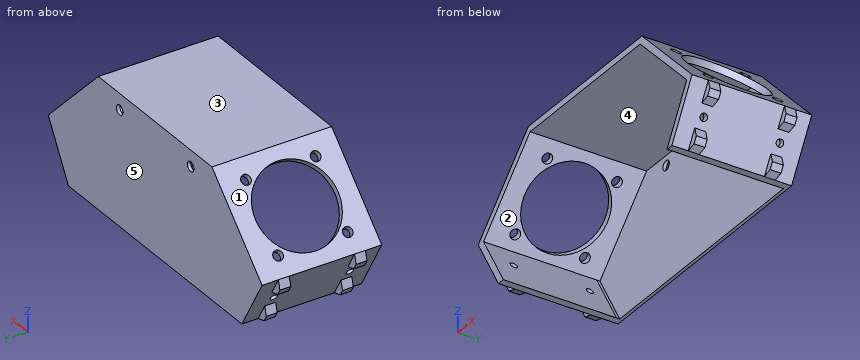
from build123d import *

# Parameters (mm, degrees)
BOSS_EXTRUDE1_DEPTH      = 55
SHELL1_T                 = -3
CUT_EXTRUDE1_REACH       = 167.077
SKETCH2_R                = 19
SKETCH2_R_2              = 2.25
CUT_EXTRUDE2_REACH       = 170.904
SKETCH3_R                = 1.65
SKETCH4_W                = 9.228601628
SKETCH4_H                = 5
BOSS_EXTRUDE2_DEPTH      = 3
CHAMFER1_SIZE            = 3
CHAMFER1_OF_MIRROR2_SIZE = 3
SKETCH5_R                = 2.25
CUT_EXTRUDE3_DEPTH       = 147.36190521
CUT_EXTRUDE4_DEPTH       = 1.5


with BuildPart() as part:
    # Sketch1 → Boss-Extrude1 (new body)
    with BuildSketch(Plane(origin=(0, 0, 0), x_dir=(1, 0, 0), z_dir=(0, 1, 0))):
        Polygon((40.050177105, -112), (-40.050177105, -112), (-75.405516164, -76.644660941), (-61.176914536, -52), (61.176914536, -52), (75.405516164, -76.644660941), align=None)
    extrude(amount=BOSS_EXTRUDE1_DEPTH)

    # Shell1
    shell1_openings = [part.faces().sort_by_distance(p)[0] for p in [
        (0, 27.5, 52),
        (0, 0, 79.968655268),
    ]]
    offset(amount=SHELL1_T, openings=shell1_openings, kind=Kind.INTERSECTION)

    # Sketch2 → Cut-Extrude1 (cut, up to next)
    with BuildSketch(Plane(origin=(76.025088553, 0, 76.025088553), x_dir=(0.7071067811865462, 0, -0.7071067811865488), z_dir=(0.7071067811865488, 0, 0.7071067811865462)), mode=Mode.PRIVATE) as cut_extrude1_sk1:
        with Locations((-25.876207674, 27.5)):
            Circle(SKETCH2_R)
    cut_extrude1_tool1 = extrude(cut_extrude1_sk1.sketch, amount=-CUT_EXTRUDE1_REACH, mode=Mode.PRIVATE) & part.part
    # Sketch2 → Cut-Extrude1 (cut, up to next)
    with BuildSketch(Plane(origin=(76.025088553, 0, 76.025088553), x_dir=(0.7071067811865462, 0, -0.7071067811865488), z_dir=(0.7071067811865488, 0, 0.7071067811865462)), mode=Mode.PRIVATE) as cut_extrude1_sk2:
        with Locations((-41.876207674, 11.5)):
            Circle(SKETCH2_R_2)
    cut_extrude1_tool2 = extrude(cut_extrude1_sk2.sketch, amount=-CUT_EXTRUDE1_REACH, mode=Mode.PRIVATE) & part.part
    # Sketch2 → Cut-Extrude1 (cut, up to next)
    with BuildSketch(Plane(origin=(76.025088553, 0, 76.025088553), x_dir=(0.7071067811865462, 0, -0.7071067811865488), z_dir=(0.7071067811865488, 0, 0.7071067811865462)), mode=Mode.PRIVATE) as cut_extrude1_sk3:
        with Locations((-9.876207674, 11.5)):
            Circle(SKETCH2_R_2)
    cut_extrude1_tool3 = extrude(cut_extrude1_sk3.sketch, amount=-CUT_EXTRUDE1_REACH, mode=Mode.PRIVATE) & part.part
    # Sketch2 → Cut-Extrude1 (cut, up to next)
    with BuildSketch(Plane(origin=(76.025088553, 0, 76.025088553), x_dir=(0.7071067811865462, 0, -0.7071067811865488), z_dir=(0.7071067811865488, 0, 0.7071067811865462)), mode=Mode.PRIVATE) as cut_extrude1_sk4:
        with Locations((-9.876207674, 43.5)):
            Circle(SKETCH2_R_2)
    cut_extrude1_tool4 = extrude(cut_extrude1_sk4.sketch, amount=-CUT_EXTRUDE1_REACH, mode=Mode.PRIVATE) & part.part
    # Sketch2 → Cut-Extrude1 (cut, up to next)
    with BuildSketch(Plane(origin=(76.025088553, 0, 76.025088553), x_dir=(0.7071067811865462, 0, -0.7071067811865488), z_dir=(0.7071067811865488, 0, 0.7071067811865462)), mode=Mode.PRIVATE) as cut_extrude1_sk5:
        with Locations((-41.876207674, 43.5)):
            Circle(SKETCH2_R_2)
    cut_extrude1_tool5 = extrude(cut_extrude1_sk5.sketch, amount=-CUT_EXTRUDE1_REACH, mode=Mode.PRIVATE) & part.part
    cut_extrude1_1 = cut_extrude1_tool1.solids().sort_by_distance((57.727847, 27.5, 94.32233))[0]
    add(cut_extrude1_1, mode=Mode.SUBTRACT)
    cut_extrude1_2 = cut_extrude1_tool2.solids().sort_by_distance((46.414138, 11.5, 105.636039))[0]
    add(cut_extrude1_2, mode=Mode.SUBTRACT)
    cut_extrude1_3 = cut_extrude1_tool3.solids().sort_by_distance((69.041555, 11.5, 83.008622))[0]
    add(cut_extrude1_3, mode=Mode.SUBTRACT)
    cut_extrude1_4 = cut_extrude1_tool4.solids().sort_by_distance((69.041555, 43.5, 83.008622))[0]
    add(cut_extrude1_4, mode=Mode.SUBTRACT)
    cut_extrude1_5 = cut_extrude1_tool5.solids().sort_by_distance((46.414138, 43.5, 105.636039))[0]
    add(cut_extrude1_5, mode=Mode.SUBTRACT)
    cut_extrude1 = cut_extrude1_1 + cut_extrude1_2 + cut_extrude1_3 + cut_extrude1_4 + cut_extrude1_5  # Cut-Extrude1 as one shape, for the pattern or mirror that repeats it

    # Sketch3 → Cut-Extrude2 (cut, up to next)
    with BuildSketch(Plane(origin=(23.366025404, 0, -13.490381057), x_dir=(-0.5000000000000074, 0, -0.8660254037844345), z_dir=(0.8660254037844344, 0, -0.5000000000000073)), mode=Mode.PRIVATE) as cut_extrude2_sk1:
        with Locations((-89.850379893, 10)):
            Circle(SKETCH3_R)
    cut_extrude2_tool1 = extrude(cut_extrude2_sk1.sketch, amount=-CUT_EXTRUDE2_REACH, mode=Mode.PRIVATE) & part.part
    # Sketch3 → Cut-Extrude2 (cut, up to next)
    with BuildSketch(Plane(origin=(23.366025404, 0, -13.490381057), x_dir=(-0.5000000000000074, 0, -0.8660254037844345), z_dir=(0.8660254037844344, 0, -0.5000000000000073)), mode=Mode.PRIVATE) as cut_extrude2_sk2:
        with Locations((-89.850379893, 45)):
            Circle(SKETCH3_R)
    cut_extrude2_tool2 = extrude(cut_extrude2_sk2.sketch, amount=-CUT_EXTRUDE2_REACH, mode=Mode.PRIVATE) & part.part
    cut_extrude2_1 = cut_extrude2_tool1.solids().sort_by_distance((68.291215, 10, 64.32233))[0]
    add(cut_extrude2_1, mode=Mode.SUBTRACT)
    cut_extrude2_2 = cut_extrude2_tool2.solids().sort_by_distance((68.291215, 45, 64.32233))[0]
    add(cut_extrude2_2, mode=Mode.SUBTRACT)
    cut_extrude2 = cut_extrude2_1 + cut_extrude2_2  # Cut-Extrude2 as one shape, for the pattern or mirror that repeats it

    # Sketch4 → Boss-Extrude2 (add)
    with BuildSketch(Plane(origin=(23.366025404, 0, -13.490381057), x_dir=(-0.5000000000000074, 0, -0.8660254037844345), z_dir=(0.8660254037844344, 0, -0.5000000000000073))):
        with Locations((-80.236079079, 10)):
            Rectangle(SKETCH4_W, SKETCH4_H)
        with Locations((-99.464680707, 10)):
            Rectangle(SKETCH4_W, SKETCH4_H)
        with Locations((-80.236079079, 45)):
            Rectangle(SKETCH4_W, SKETCH4_H)
        with Locations((-99.464680707, 45)):
            Rectangle(SKETCH4_W, SKETCH4_H)
    boss_extrude2 = extrude(amount=BOSS_EXTRUDE2_DEPTH)

    # Chamfer1
    chamfer1_edges = [part.edges().sort_by_distance(p)[0] for p in [
        (63.774990748, 10, 50.5),
        (63.774990748, 45, 50.5),
        (68.389291562, 45, 58.492203451),
        (68.389291562, 10, 58.492203451),
        (73.389291562, 10, 67.152457489),
        (73.389291562, 45, 67.152457489),
        (78.003592376, 10, 75.144660941),
        (78.003592376, 45, 75.144660941),
    ]]
    chamfer(chamfer1_edges, length=CHAMFER1_SIZE - 0.0001)  # a hair under: the kernel refuses the full size

    # Mirror2: Cut-Extrude1, Cut-Extrude2, Boss-Extrude2 across plane
    add(cut_extrude1.mirror(Plane(origin=(0, 0, 0), x_dir=(0, 0, 1), z_dir=(1, 0, 0))), mode=Mode.SUBTRACT)
    add(cut_extrude2.mirror(Plane(origin=(0, 0, 0), x_dir=(0, 0, 1), z_dir=(1, 0, 0))), mode=Mode.SUBTRACT)
    add(boss_extrude2.mirror(Plane(origin=(0, 0, 0), x_dir=(0, 0, 1), z_dir=(1, 0, 0))))

    # Chamfer1 of Mirror2
    chamfer1_of_mirror2_edges = [part.edges().sort_by_distance(p)[0] for p in [
        (-63.774990748, 10, 50.5),
        (-63.774990748, 45, 50.5),
        (-68.389291562, 45, 58.492203451),
        (-68.389291562, 10, 58.492203451),
        (-73.389291562, 10, 67.152457489),
        (-73.389291562, 45, 67.152457489),
        (-78.003592376, 10, 75.144660941),
        (-78.003592376, 45, 75.144660941),
    ]]
    chamfer(chamfer1_of_mirror2_edges, length=CHAMFER1_OF_MIRROR2_SIZE - 0.0001)  # a hair under: the kernel refuses the full size

    # Sketch5 → Cut-Extrude3 (cut, through all)
    with BuildSketch(Plane(origin=(0, 55, 0), x_dir=(1, 0, 0), z_dir=(0, 1, 0))):
        with Locations(Location((-25, -104.5, 0), (0, 0, 270))):
            Circle(SKETCH5_R)
        with Locations(Location((25, -104.5, 0), (0, 0, 270))):
            Circle(SKETCH5_R)
    extrude(amount=-CUT_EXTRUDE3_DEPTH, mode=Mode.SUBTRACT)

    # Sketch6 → Cut-Extrude4 (cut)
    with BuildSketch(Plane.XZ.offset(-52)):
        Polygon((-57.712812921, 52), (57.712812921, 52), (71.656449471, 76.151086947), (38.807536418, 109), (-38.807536418, 109), (-71.656449471, 76.151086947), align=None)
    extrude(amount=-CUT_EXTRUDE4_DEPTH, mode=Mode.SUBTRACT)


solid = part.part
Check sheet for the modelled part. Datum: model origin and axes. Units: mm. Face numbers are marked on the shaded views. A direction names the side the tool comes from. Give positions to 0.01 mm unless a question says otherwise; leave off trailing zeros. Order: outer loops, then holes, each group sorted by start corner. A loop starts at its lowest first (then second) coordinate and runs counter-clockwise, first axis right, second up. Notation, with made-up numbers: (31.5, -32) - (82.5, -32) arc R19 ccw to (82.5, 2) - close; hole circle Ø1 at (75, 58). An arc over 180 degrees is marked (long way). Answer as CSV lines item,"result".
1. Section check D-D (y = 26). Record the boundary of the cut face in (x, z), then the cut area to 3 significant figures.
Result sheet:
outline,"(-75.41, 76.64) - (-61.18, 52) - (-57.71, 52) - (-71.66, 76.15) - (-69, 78.81) - (-71.12, 80.93) - close; (-44.33, 107.72) - (-42.21, 105.59) - (-38.81, 109) - (38.81, 109) - (42.21, 105.59) - (44.33, 107.72) - (40.05, 112) - (-40.05, 112) - close; (57.71, 52) - (61.18, 52) - (75.41, 76.64) - (71.12, 80.93) - (69, 78.81) - (71.66, 76.15) - close"
area,"468 mm²"
2. Section check B-B (y = 16). Record the boundary of the cut face in (x, z).
Result sheet:
outline,"(-75.41, 76.64) - (-61.18, 52) - (-57.71, 52) - (-71.66, 76.15) - (-66.3, 81.51) - (-68.42, 83.63) - close; (-47.03, 105.02) - (-44.91, 102.9) - (-38.81, 109) - (38.81, 109) - (44.91, 102.9) - (47.03, 105.02) - (40.05, 112) - (-40.05, 112) - close; (57.71, 52) - (61.18, 52) - (75.41, 76.64) - (68.42, 83.63) - (66.3, 81.51) - (71.66, 76.15) - close"
3. Section check A-A (x = 25). Record the boundary of the cut face in (y, z), then the cut area to 3 significant figures.
Result sheet:
outline,"(0, 109) - (53.5, 109) - (53.5, 106.75) - (55, 106.75) - (55, 112) - (0, 112) - close; (53.5, 52) - (55, 52) - (55, 102.25) - (53.5, 102.25) - close"
area,"244 mm²"
4. Go/stop test with flat-tipped pins: P1, Ø12, axis at x = -57, z = 67, coming from the -Y side; P2, Ø4.5, axis at x = -65, z = 54, coming from the +Y side; P3, Ø4, axis at x = 4, y = 28.5, coming from the -Z side. Record where each tip stops, or that it passes through.
Result sheet:
P1,"y = 53.5"
P2,"y = 47.5"
P3,"z = 109"
5. Mould release check, pull along X, two halves, no side actions. Record for the marked faces 1, 2 and 3: released by +X, released by -X, zero draft, split by the parting line, or undercut.
Result sheet:
face 1,"released by -X"
face 2,"undercut"
face 3,"zero draft"
6. Tool access check on the marked faces 4 and 5. Record the directions out of +Z, -Z, +X, -X, +Y, -Y that give a thin tool (end or side, any length) a straight path to the whole face; none if there is none.
Result sheet:
face 4,"-Z, -Y"
face 5,"+Z, -Z, +X, -X, +Y"
7. Section check C-C (z = 90). State how many separate pieces and enclosed holes the cut face has, then the cut area to 3 significant figures.
Result sheet:
separate pieces,"3"
enclosed holes,"0"
area,"328 mm²"
8. Scan lines: probe 1 along X at (y, z) = (54.3, 104.5); probe 2 along X at (y, z) = (54, 104); probe 3 along Y at (x, z) = (58, 59). Record each from-to range of solid material in increasing order. Write a range as from..to.
Result sheet:
probe 1,"-47.55..-27.25, -22.75..22.75, 27.25..47.55"
probe 2,"-48.05..-27.19, -22.81..22.81, 27.19..48.05"
probe 3,"53.5..55"
